from build123d import *

# Parameters (mm, degrees)
SKETCH1_W                = 8
SKETCH1_H                = 6.87
BOSS_EXTRUDE3_DEPTH      = 8
SKETCH2_W                = 8
SKETCH2_H                = 14.87
BOSS_EXTRUDE5_DEPTH      = 12.93
M1_2X0_25_TAPPED_HOLE1_D = 0.95
F_1_0MM_DOWEL_HOLE1_D    = 6


with BuildPart() as part:
    # Sketch1 → Boss-Extrude3 (new body)
    with BuildSketch(Plane(origin=(0, 0, 0), x_dir=(1, 0, 0), z_dir=(0, 1, 0))):
        with Locations((-14.308724832, -6.420704698)):
            Rectangle(SKETCH1_W, SKETCH1_H)
    extrude(amount=BOSS_EXTRUDE3_DEPTH)

    # Sketch2 → Boss-Extrude5 (add)
    with BuildSketch(Plane(origin=(0, 8, 0), x_dir=(1, 0, 0), z_dir=(0, 1, 0))):
        with Locations((-14.308724832, -10.420704698)):
            Rectangle(SKETCH2_W, SKETCH2_H)
    extrude(amount=BOSS_EXTRUDE5_DEPTH)

    # M1.2x0.25 Tapped Hole1 (through all)
    with Locations(Plane(origin=(0, 20.93, 0), x_dir=(1, 0, 0), z_dir=(0, 1, 0))):
        with Locations((-17.308724832, -11.855704698), (-11.308724832, -11.855704698), (-17.308724832, -16.855704698), (-11.308724832, -16.855704698)):
            Hole(M1_2X0_25_TAPPED_HOLE1_D / 2)

    # Ø1.0mm Dowel Hole1 (through all)
    with Locations(Plane(origin=(0, 0, 2.985704698), x_dir=(-1, 0, 0), z_dir=(0, 0, -1))):
        with Locations((14.308724832, 4)):
            Hole(F_1_0MM_DOWEL_HOLE1_D / 2)


solid = part.part
Could you check a few things on this model? Use its own coordinates, in mm. A direction names the side the tool comes from. Round coordinates to 2 decimals unless told otherwise and drop trailing zeros. Order: outer loops, then holes, each group sorted by start corner. A loop starts at its lowest first (then second) coordinate and runs counter-clockwise, first axis right, second up.
(1) Imagine slicing it at C-C (z = 8.75). Write out the boundary of the cut face in (x, y), plus the area to 3 significant figures.
Response values:
outline: (-18.31, 0) - (-10.31, 0) - (-10.31, 20.93) - (-18.31, 20.93) - close; hole circle Ø6 at (-14.31, 4)
area: 139 mm2
(2) Imagine slicing it at B-B (x = -12.75). Write out the boundary of the cut face in (y, z), plus the area to 3 significant figures.
Response values:
outline: (0, 2.99) - (1.44, 2.99) - (1.44, 9.86) - (0, 9.86) - close; (6.56, 2.99) - (20.93, 2.99) - (20.93, 17.86) - (8, 17.86) - (8, 9.86) - (6.56, 9.86) - close
area: 212 mm2
(3) If we mould it in two halves opening along Z, with no side actions, what happens to faces 1 (the cylindrical face through (-11.748, 14.374, 17.038)), 2 (the flat face through (-14, 13, 2.986)), 3 (the flat face through (-17, 6, 9.856)), 4 (the cylindrical face through (-11.54, 2.85, 6.47))? For each: released by +Z, released by -Z, zero draft, split by the parting line, or undercut.
Response values:
face 1: undercut
face 2: released by -Z
face 3: released by +Z
face 4: zero draft
(4) Please list where these lines run through material, in increasing order: line 1 along Z through (x, y) = (-11.25, 17.5); line 2 along Z through (x, y) = (-12.25, 7.75); line 3 along Y through (x, z) = (-12.25, 9).
Response values:
line 1: z = 2.99 to 11.38, 12.33 to 16.38, 17.33 to 17.86
line 2: z = 2.99 to 9.86
line 3: y = 0 to 1.82, 6.18 to 20.93
(5) Which directions (+Z, -Z, +X, -X, +Y, -Y) give clear straight access to the entire face, cutting with the end or side of a thin tool? Please do faces 5 (the flat face through (-14, 0, 6)), 6 (the flat face through (-14, 8, 14)).
Response values:
face 5: +Z, -Z, +X, -X, -Y
face 6: +Z, +X, -X, -Y
(6) I'm going to push flat-ended pins straight in: pin 1 (3 mm diameter, centred on x = -15, z = 8, fed in from -Y); pin 2 (4 mm diameter, centred on x = -15.5, y = 2, fed in from +Z); pin 3 (4 mm diameter, centred on x = -15, z = 13, fed in from -Y). Where does each tip first touch, or does it pass through?
Response values:
pin 1: stops at y = 0
pin 2: stops at z = 9.86
pin 3: stops at y = 8
(7) Imagine slicing it at A-A (y = 4). Write out the boundary of the cut face in (x, z), plus the area to 3 significant figures.
Response values:
outline: (-18.31, 2.99) - (-17.31, 2.99) - (-17.31, 9.86) - (-18.31, 9.86) - close; (-11.31, 2.99) - (-10.31, 2.99) - (-10.31, 9.86) - (-11.31, 9.86) - close
area: 13.7 mm2
(8) Imagine slicing it at D-D (y = 11). Write out the boundary of the cut face in (x, z) (3 decimals).
Response values:
outline: (-18.309, 2.986) - (-10.309, 2.986) - (-10.309, 17.856) - (-18.309, 17.856) - close; hole circle Ø0.95 at (-17.309, 11.856); hole circle Ø0.95 at (-17.309, 16.856); hole circle Ø0.95 at (-11.309, 11.856); hole circle Ø0.95 at (-11.309, 16.856)
